Verification items for the finished model (mm, model axes). Face numbers are marked on the shaded views. Round coordinates to 2 decimals unless told otherwise and drop trailing zeros. Write each loop counter-clockwise with the first axis right and the second up, starting at its lowest first coordinate (ties: lowest second). Pieces come first, ordered by that corner, then holes. Notation, with made-up numbers: (75.5, 86) - (91.5, 86) arc R24 ccw to (91.5, 99) - close; hole circle Ø6 at (4.25, -6.75). An arc over 180 degrees is marked (long way). Answer as a JSON object with one key per item and string values. Group by question number.
1) Go/stop test with a flat-tipped pin: pin 1 Ø5 at (x, y) = (102.5, -2) entering from +Z. Record where the tip stops, or that it passes through.
2) Thickness scan on line 1 (Y direction, x = 101.6, z = 4); line 2 (Y direction, x = 101.6, z = 1.1); line 3 (X direction, y = 0.5, z = 4.15). Record the ranges inside material, lowest first.
3) Mould release check, pull along Z, two halves, no side actions. Record for the marked faces 1 and 2: +Z half, -Z half, draft (parallel to the pull), parting line (faces both ways), or undercut.
4) Section check B-B (z = 3.8). Enter the section's corners in (x, y) (1 decimal), then the cut area to 3 significant figures.
5) Section check A-A (y = 0). Enter the section's corners in (x, z).
6) Section check C-C (x = 12.7). Enter the section's corners in (y, z).
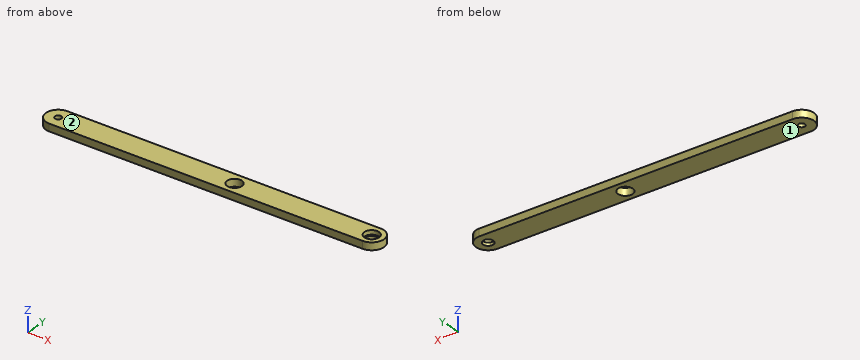
```python
from build123d import *

# Parameters (mm, degrees)
SKETCH1_R                 = 4.7625
BOSS_EXTRUDE1_DEPTH       = 4.7625
SKETCH1_3_R               = 4.7625
SKETCH1_3_R_2             = 3.3734375
BOSS_EXTRUDE2_DEPTH       = 2.032
M5X0_8_TAPPED_HOLE1_D     = 4.2
M5X0_8_TAPPED_HOLE1_DEPTH = 11.1333927
M5X0_8_TAPPED_HOLE1_TIP   = 1.2618073


with BuildPart() as part:
    # Sketch1 → Boss-Extrude1 (new body)
    with BuildSketch(Plane.XY):
        with BuildLine():
            Line((-101.6, 7.9375), (101.6, 7.9375))
            ThreePointArc((101.6, 7.9375), (109.5375, 0), (101.6, -7.9375))
            Line((101.6, -7.9375), (-101.6, -7.9375))
            ThreePointArc((-101.6, -7.9375), (-109.5375, 0), (-101.6, 7.9375))
        make_face()
        with Locations(Location((101.6, 0, 0), (0, 0, 180))):
            Circle(SKETCH1_R, mode=Mode.SUBTRACT)
        with Locations(Location((12.7, 0, 0), (0, 0, 180))):
            Circle(SKETCH1_R, mode=Mode.SUBTRACT)
    extrude(amount=BOSS_EXTRUDE1_DEPTH)

    # Sketch1_3 → Boss-Extrude2 (add)
    with BuildSketch(Plane.XY):
        with Locations(Location((101.6, 0, 0), (0, 0, 180))):
            Circle(SKETCH1_3_R)
        with Locations((101.6, 0)):
            Circle(SKETCH1_3_R_2, mode=Mode.SUBTRACT)
    extrude(amount=BOSS_EXTRUDE2_DEPTH)

    # M5x0.8 Tapped Hole1
    with Locations(Plane.XY.offset(4.7625)):
        with Locations((-101.6, 0)):
            Hole(M5X0_8_TAPPED_HOLE1_D / 2, depth=M5X0_8_TAPPED_HOLE1_DEPTH)
            with Locations((0, 0, -(M5X0_8_TAPPED_HOLE1_DEPTH + M5X0_8_TAPPED_HOLE1_TIP / 2))):  # 118° drill point
                Cone(0, M5X0_8_TAPPED_HOLE1_D / 2, M5X0_8_TAPPED_HOLE1_TIP, mode=Mode.SUBTRACT)


solid = part.part
```
Returned:
{
 "1": {"pin 1": "z = 2.03"},
 "2": {"line 1": "-7.94 to -4.76, 4.76 to 7.94", "line 2": "-7.94 to -3.37, 3.37 to 7.94", "line 3": "-109.52 to -103.64, -99.56 to 7.96, 17.44 to 96.86, 106.34 to 109.52"},
 "3": {"face 1": "-Z half", "face 2": "+Z half"},
 "4": {"outline": "(-101.6, -7.9) - (101.6, -7.9) arc R7.9 ccw to (101.6, 7.9) - (-101.6, 7.9) arc R7.9 ccw to start; hole circle Ø4.2 at (-101.6, 0); hole circle Ø9.5 at (12.7, 0); hole circle Ø9.5 at (101.6, 0)", "area": "3,270 mm2"},
 "5": {"outline": "(-109.54, 0) - (-103.7, 0) - (-103.7, 4.76) - (-109.54, 4.76) - close; (-99.5, 0) - (7.94, 0) - (7.94, 4.76) - (-99.5, 4.76) - close; (17.46, 0) - (98.23, 0) - (98.23, 2.03) - (96.84, 2.03) - (96.84, 4.76) - (17.46, 4.76) - close; (104.97, 0) - (109.54, 0) - (109.54, 4.76) - (106.36, 4.76) - (106.36, 2.03) - (104.97, 2.03) - close"},
 "6": {"outline": "(-7.94, 0) - (-4.76, 0) - (-4.76, 4.76) - (-7.94, 4.76) - close; (4.76, 0) - (7.94, 0) - (7.94, 4.76) - (4.76, 4.76) - close"}
}
